Verification items for the finished model (mm, model axes). Coordinates: 2 decimals unless noted, no trailing zeros. Loops run counter-clockwise (first coordinate to the right, second up) from the corner with the lowest first, then second, coordinate; pieces in that order, holes last. Notation, with made-up numbers: (-8, -6) - (49, -6) arc R26 cw to (49, 24) - close; hole circle Ø11 at (38, -14). An arc over 180 degrees is marked (long way). One line per item, written item: value. Start each with the question number.
(1) Draft check along Z on faces 1 (the face through (-1, 1.6, -1)), 2 (the face through (43.023, 0.789, -57.368)), 3 (the face through (-39.45, 0.79, -57.37)). Enter one of: +Z half, -Z half, draft (parallel to the pull), parting line (faces both ways), or undercut.
(2) Thickness scan on probe 1 along Z at (x, y) = (41, 1.3); probe 2 along Z at (x, y) = (15.5, 1.35); probe 3 along Z at (x, y) = (-40, 1.05). Record the ranges inside material, lowest first. Write a range as [from, to].
(3) Section check A-A (y = 1.3). Record the boundary of the cut face in (x, z).
(4) Section check B-B (x = -15). Record the boundary of the cut face in (y, z), plus the area to 3 significant figures.
(5) Gauge pin test, flat end, axial feed: P1, Ø0.5, axis at x = -5, y = 1, coming from the +Z side. Record the tip position at first contact, or that the pin passes through.
```python
from build123d import *

# Parameters (mm, degrees)
SKETCH1_W                = 92
SKETCH1_H                = 127
BOSS_EXTRUDE1_DEPTH      = 1.6
M4_CLEARANCE_HOLE1_D     = 4.5
M4_CLEARANCE_HOLE1_DEPTH = 50
M4_CLEARANCE_HOLE1_TIP   = 1.351936393
SKETCH4_W                = 55
SKETCH4_H                = 10
CUT_EXTRUDE1_DEPTH       = 1.6
FILLET1_R                = 2.032


with BuildPart() as part:
    # Sketch1 → Boss-Extrude1 (new body)
    with BuildSketch(Plane(origin=(0, 0, 0), x_dir=(1, 0, 0), z_dir=(0, 1, 0))):
        Rectangle(SKETCH1_W, SKETCH1_H)
    extrude(amount=BOSS_EXTRUDE1_DEPTH)

    # M4 Clearance Hole1
    with Locations(Plane(origin=(0, 1.6, 0), x_dir=(1, 0, 0), z_dir=(0, 1, 0))):
        with Locations((-41.2375, 58.7375), (41.2375, 58.7375), (41.2375, -58.7375), (-41.2375, -58.7375)):
            Hole(M4_CLEARANCE_HOLE1_D / 2, depth=M4_CLEARANCE_HOLE1_DEPTH)
            with Locations((0, 0, -(M4_CLEARANCE_HOLE1_DEPTH + M4_CLEARANCE_HOLE1_TIP / 2))):  # 118° drill point
                Cone(0, M4_CLEARANCE_HOLE1_D / 2, M4_CLEARANCE_HOLE1_TIP, mode=Mode.SUBTRACT)

    # Sketch4 → Cut-Extrude1 (cut)
    with BuildSketch(Plane(origin=(0, 1.6, 0), x_dir=(1, 0, 0), z_dir=(0, 1, 0))):
        with Locations((0, -58.5)):
            Rectangle(SKETCH4_W, SKETCH4_H)
    extrude(amount=-CUT_EXTRUDE1_DEPTH, mode=Mode.SUBTRACT)

    # Fillet1
    fillet1_edges = [part.edges().sort_by_distance(p)[0] for p in [
        (27.5, 0.8, 53.5),
        (27.5, 0.8, 63.5),
        (-27.5, 0.8, 63.5),
        (-27.5, 0.8, 53.5),
        (46, 0.8, 63.5),
        (-46, 0.8, 63.5),
        (-46, 0.8, -63.5),
        (46, 0.8, -63.5),
    ]]
    fillet(fillet1_edges, radius=FILLET1_R)


solid = part.part
```
Responses:
1. face 1: draft
1. face 2: undercut
1. face 3: undercut
2. probe 1: z = [-63.5, -60.97], [-56.5, 56.5], [60.97, 63.5]
2. probe 2: z = [-63.5, 53.5]
2. probe 3: z = [-63.5, -60.62], [-56.86, 56.86], [60.62, 63.5]
3. outline: (-46, -61.47) arc R2.03 ccw to (-43.97, -63.5) - (43.97, -63.5) arc R2.03 ccw to (46, -61.47) - (46, 61.47) arc R2.03 ccw to (43.97, 63.5) - (29.53, 63.5) arc R2.03 ccw to (27.5, 61.47) - (27.5, 55.53) arc R2.03 cw to (25.47, 53.5) - (-25.47, 53.5) arc R2.03 cw to (-27.5, 55.53) - (-27.5, 61.47) arc R2.03 ccw to (-29.53, 63.5) - (-43.97, 63.5) arc R2.03 ccw to (-46, 61.47) - close; hole circle Ø4.5 at (-41.24, -58.74); hole circle Ø4.5 at (-41.24, 58.74); hole circle Ø4.5 at (41.24, -58.74); hole circle Ø4.5 at (41.24, 58.74)
4. outline: (0, -63.5) - (1.6, -63.5) - (1.6, 53.5) - (0, 53.5) - close
4. area: 187 mm²
5. P1: stops at z = 53.5
